For this review, take the finished solid that the model builds, in its own axes (mm). Face numbers are marked on the shaded views. A direction names the side the tool comes from. Give positions to 0.01 mm unless a question says otherwise; leave off trailing zeros. Loops run counter-clockwise (first coordinate to the right, second up) from the corner with the lowest first, then second, coordinate; pieces in that order, holes last.
```python
from build123d import *

# Parameters (mm, degrees)
SKETCH_1_W          = 936
SKETCH_1_H          = 736
SKETCH_1_W_2        = 900
SKETCH_1_H_2        = 700
EXTRUDE_1_DEPTH     = 400
SKETCH_2_W          = 776
SKETCH_2_H          = 280
CUT_EXTRUDE_1_DEPTH = 179


with BuildPart() as part:
    # 草图1 → 凸台-拉伸1 (new body)
    with BuildSketch(Plane(origin=(0, 0, 0), x_dir=(1, 0, 0), z_dir=(0, 1, 0))):
        with Locations((473.076923077, -350)):
            Rectangle(SKETCH_1_W, SKETCH_1_H)
        with Locations((473.076923077, -350)):
            Rectangle(SKETCH_1_W_2, SKETCH_1_H_2, mode=Mode.SUBTRACT)
    extrude(amount=EXTRUDE_1_DEPTH)

    # 草图2 → 切除-拉伸1 (cut)
    with BuildSketch(Plane.XY.offset(718)):
        with Locations((473.076923077, 200)):
            Rectangle(SKETCH_2_W, SKETCH_2_H)
    extrude(amount=-CUT_EXTRUDE_1_DEPTH, mode=Mode.SUBTRACT)


solid = part.part
```
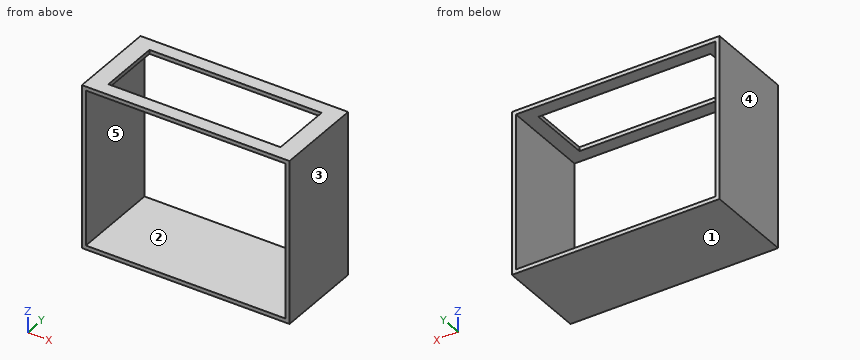
Item 1: Tool access review of the marked faces 4 and 5: name each direction out of +Z, -Z, +X, -X, +Y, -Y from which nothing blocks a thin tool from reaching the whole face with its end or side.
Answer:
face 4: +Z, -Z, -X, +Y, -Y
face 5: +Y, -Y
Item 2: Take a section at B-B on z = 147. Give the boundary of the cut face in (x, y).
Answer:
outline: (5.08, 0) - (23.08, 0) - (23.08, 400) - (5.08, 400) - close; (923.08, 0) - (941.08, 0) - (941.08, 400) - (923.08, 400) - close
Item 3: Take a section at A-A on x = 170. Give the boundary of the cut face in (y, z), and give its area (3 significant figures).
Answer:
outline: (0, -18) - (400, -18) - (400, 0) - (0, 0) - close; (0, 700) - (60, 700) - (60, 718) - (0, 718) - close; (340, 700) - (400, 700) - (400, 718) - (340, 718) - close
area: 9,360 mm2
Item 4: For L1, parallel to X at y = 174.5, z = 465.5; L2, parallel to Z at x = 257.5, y = 152; L3, parallel to Z at x = 117, y = 44, list the stretches that pass through material, from the lowest coordinate up.
Answer:
L1: x = 5.08 to 23.08, 923.08 to 941.08
L2: z = -18 to 0
L3: z = -18 to 0, 700 to 718
Item 5: The part is to be moulded in two halves that separate along Z. For the marked faces 1, 2 and 3, say which applies: released by +Z, released by -Z, zero draft, split by the parting line, or undercut.
Answer:
face 1: released by -Z
face 2: undercut
face 3: zero draft
Item 6: Take a section at C-C on y = 235. Give the boundary of the cut face in (x, z), and give its area (3 significant figures).
Answer:
outline: (5.08, -18) - (941.08, -18) - (941.08, 718) - (861.08, 718) - (861.08, 700) - (923.08, 700) - (923.08, 0) - (23.08, 0) - (23.08, 700) - (85.08, 700) - (85.08, 718) - (5.08, 718) - close
area: 44,900 mm2
Item 7: Clearance check with a flat-ended pin moving along its axis: pin 1 Ø5 at (x, y) = (535.5, 95.5) entering from +Z. State where the tip first meets the part, or that it passes through.
Answer:
pin 1: stops at z = 0
